from build123d import *

# Parameters (mm, degrees)
MODEL_R             = 1.2
BOSS_EXTRUDE1_DEPTH = 12.4


with BuildPart() as part:
    # Model → Boss-Extrude1 (new body)
    with BuildSketch(Plane.XY):
        with BuildLine():
            Line((47.4, 0), (52.4, 0))
            Line((52.4, 0), (52.4, 52.4))
            Line((52.4, 52.4), (13, 52.4))
            ThreePointArc((13, 52.4), (10.878679656, 51.521320344), (10, 49.4))
            Line((10, 49.4), (10, 35.4))
            ThreePointArc((10, 35.4), (9.121320344, 33.278679656), (7, 32.4))
            Line((7, 32.4), (3, 32.4))
            ThreePointArc((3, 32.4), (0.878679656, 31.521320344), (0, 29.4))
            Line((0, 29.4), (0, 0))
            Line((0, 0), (10, 0))
            Line((10, 0), (10, 12.4))
            Line((10, 12.4), (30, 12.4))
            Line((30, 12.4), (30, 42.4))
            Line((30, 42.4), (42.4, 42.4))
            Line((42.4, 42.4), (42.4, 12.4))
            Line((42.4, 12.4), (47.4, 12.4))
            Line((47.4, 12.4), (47.4, 0))
        make_face()
        with Locations(Location((42.4, 47.4, 0), (0, 0, 180))):
            Circle(MODEL_R, mode=Mode.SUBTRACT)
    extrude(amount=BOSS_EXTRUDE1_DEPTH)


solid = part.part
Check sheet for the modelled part. Datum: model origin and axes. Units: mm. A direction names the side the tool comes from. Give positions to 0.01 mm unless a question says otherwise; leave off trailing zeros. Order: outer loops, then holes, each group sorted by start corner. A loop starts at its lowest first (then second) coordinate and runs counter-clockwise, first axis right, second up. Notation, with made-up numbers: M 67,38 L 120,38 A18 ccw 120,56 Z; hole C -8,26.5 d1. An arc over 180 degrees is marked long. Answer as CSV lines item,"result". Start each with the question number.
Item 1: Cross-section at C-C on y = 37.5. Enter the section's corners in (x, z).
Item 2: Thickness scan on line 1 (X direction, y = 3, z = 6); line 2 (X direction, y = 37, z = 3.5); line 3 (Y direction, x = 21, z = 2.25). Record the ranges inside material, lowest first. Write a range as [from, to].
Item 3: Cross-section at B-B on y = 5. Enter the section's corners in (x, z), plus the area to 3 significant figures.
Item 4: Mould release check, pull along X, two halves, no side actions. Record for faces 4 (the face through (26, 27, 12.4)), 5 (the face through (20, 12.4, 6)), 6 (the face through (0.9, 31.54, 6.11)): +X half, -X half, draft (parallel to the pull), parting line (faces both ways), or undercut.
Item 5: Gauge pin test, flat ends, axial feed: P1, Ø3.5, axis at x = 22.5, z = 5, coming from the -Y side; P2, Ø2, axis at x = 42.4, y = 47.4, coming from the -Z side; P3, Ø6, axis at y = 43, z = 5, coming from the -X side; P4, Ø1.2, axis at x = 5.5, z = 8, coming from the +Y side. Record the tip position at first contact, or that the pin passes through.
Item 6: Cross-section at A-A on z = 4.75. Enter the section's corners in (x, y).
Item 7: Tool access check on faces 1 (the face through (50, 0, 6)), 2 (the face through (10, 42, 6)), 3 (the face through (36, 42.4, 6)). Record the directions out of +Z, -Z, +X, -X, +Y, -Y that give a thin tool (end or side, any length) a straight path to the whole face; none if there is none.
Item 8: Cross-section at D-D on x = 33.5. Enter the section's corners in (y, z).
Established:
1,outline,"M 10,0 L 30,0 L 30,12.4 L 10,12.4 Z; M 42.4,0 L 52.4,0 L 52.4,12.4 L 42.4,12.4 Z"
2,line 1,"x = [0, 10], [47.4, 52.4]"
2,line 2,"x = [10, 30], [42.4, 52.4]"
2,line 3,"y = [12.4, 52.4]"
3,outline,"M 0,0 L 10,0 L 10,12.4 L 0,12.4 Z; M 47.4,0 L 52.4,0 L 52.4,12.4 L 47.4,12.4 Z"
3,area,"186 mm^2"
4,face 4,"draft"
4,face 5,"undercut"
4,face 6,"-X half"
5,P1,"stops at y = 12.4"
5,P2,"passes through"
5,P3,"stops at x = 10"
5,P4,"stops at y = 32.4"
6,outline,"M 0,0 L 10,0 L 10,12.4 L 30,12.4 L 30,42.4 L 42.4,42.4 L 42.4,12.4 L 47.4,12.4 L 47.4,0 L 52.4,0 L 52.4,52.4 L 13,52.4 A3 ccw 10,49.4 L 10,35.4 A3 cw 7,32.4 L 3,32.4 A3 ccw 0,29.4 Z; hole C 42.4,47.4 d2.4"
7,face 1,"+Z, -Z, +X, -X, -Y"
7,face 2,"+Z, -Z, -X, +Y"
7,face 3,"+Z, -Z, -Y"
8,outline,"M 42.4,0 L 52.4,0 L 52.4,12.4 L 42.4,12.4 Z"
